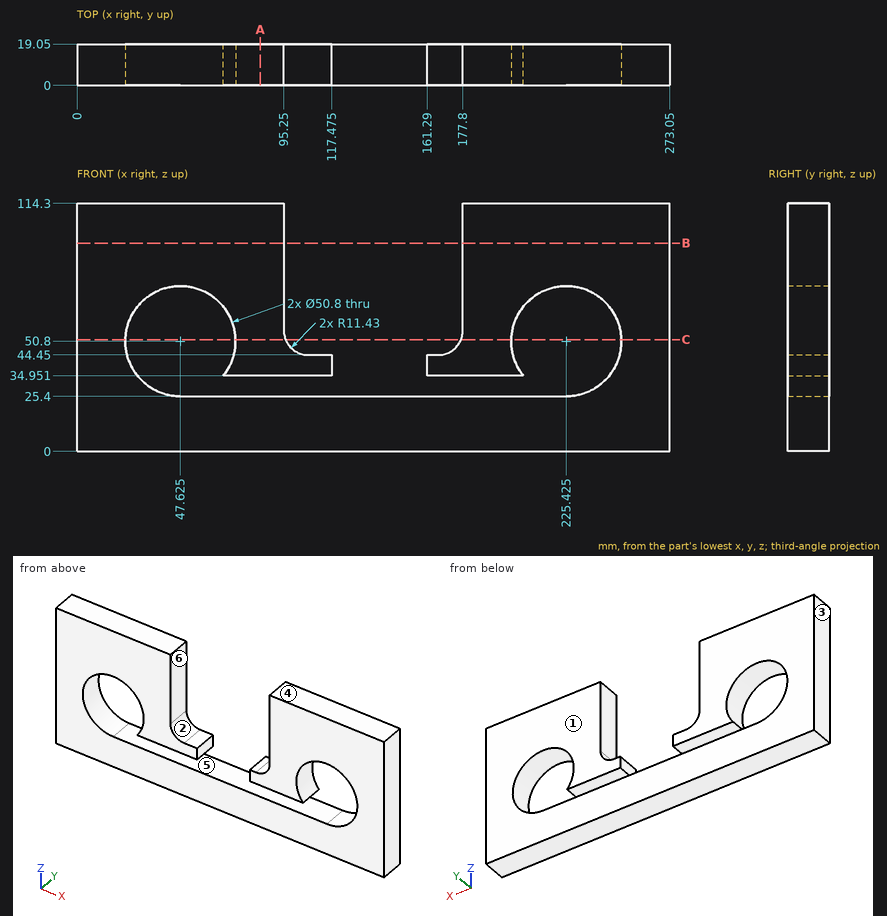
Print and shaded views of the part. All mm, measured from the part's lowest x, y and z. A direction names the side the tool comes from. Coordinates: 2 decimals unless noted, no trailing zeros. Order: outer loops, then holes, each group sorted by start corner. A loop starts at its lowest first (then second) coordinate and runs counter-clockwise, first axis right, second up. Notation, with made-up numbers: M 22.5,6 L 61.5,6 A20 ccw 61.5,30 Z; hole C -3.75,-15 d1. An arc over 180 degrees is marked long. Write each question's results on one line, items separated by ' | '. Start each with the question number.
Q1. Cut at B-B (z = 96). List the corners of the cut face in (x, y), then the cut area to 3 significant figures.
Q2. Cut at C-C (z = 51.5). List the corners of the cut face in (x, y).
Q3. Cut at A-A (x = 84.5). List the corners of the cut face in (y, z).
Q4. Drill centre lines: probe 1 along X at (y, z) = (4.25, 82); probe 2 along X at (y, z) = (14, 46.5); probe 3 along Z at (x, y) = (192.5, 2.75). Where is each one in solid material? Low to high. Write a range as from..to.
Q5. Flat gauge pin, fed straight in: P1, Ø5.5, axis at x = 111, y = 8, coming from the +Z side. Where does the tip first touch, or does it go through?
Q6. Which spindle directions (+Z, -Z, +X, -X, +Y, -Y) get a long thin tool onto all of the face, cutting with end or side? Do the marked faces 4, 5 and 6. Say none if no direction does.
Q7. Pull direction X, two halves, no side cores. Call the marked faces 1, 2 and 3: +X half, -X half, draft (parallel to the pull), parting line (faces both ways), or undercut.
Found:
1) outline: M 0,0 L 95.25,0 L 95.25,19.05 L 0,19.05 Z; M 177.8,0 L 273.05,0 L 273.05,19.05 L 177.8,19.05 Z | area: 3,630 mm²
2) outline: M 0,0 L 22.23,0 L 22.23,19.05 L 0,19.05 Z; M 73.02,0 L 96.12,0 L 96.12,19.05 L 73.02,19.05 Z; M 176.93,0 L 200.03,0 L 200.03,19.05 L 176.93,19.05 Z; M 250.82,0 L 273.05,0 L 273.05,19.05 L 250.82,19.05 Z
3) outline: M 0,0 L 19.05,0 L 19.05,25.4 L 0,25.4 Z; M 0,34.95 L 19.05,34.95 L 19.05,114.3 L 0,114.3 Z
4) probe 1: 0..95.25, 177.8..273.05 | probe 2: 0..22.59, 72.66..100.15, 172.9..200.39, 250.46..273.05 | probe 3: 0..25.4, 34.95..114.3
5) P1: z = 44.45
6) face 4: +Z, +X, -X, +Y, -Y | face 5: +Y, -Y | face 6: +Z, +Y, -Y
7) face 1: draft | face 2: undercut | face 3: -X half
